Check sheet for the modelled part. Datum: model origin and axes. Units: mm. Face numbers are marked on the shaded views. A direction names the side the tool comes from. Coordinates: 2 decimals unless noted, no trailing zeros. Order: outer loops, then holes, each group sorted by start corner. A loop starts at its lowest first (then second) coordinate and runs counter-clockwise, first axis right, second up.
1. Cross-section at B-B (z = 8.5). Enter the section's corners in (x, y).
2. Cross-section at A-A (z = 43.5). Enter the section's corners in (x, y), then the cut area to 3 significant figures.
3. Thickness scan on line 1 (X direction, y = 0, z = 46.75); line 2 (Y direction, x = 0, z = 48.5); line 3 (Z direction, x = 1.2, y = 2.25). Record the ranges inside material, lowest first.
4. Set-up check for the marked faces 1 and 2: record each of +Z, -Z, +X, -X, +Y, -Y from which the full face is reachable in a straight line by a thin tool's end or side.
5. Gauge pin test, flat ends, axial feed: pin 1 Ø1.5 at (x, y) = (0, 0) entering from +Z; pin 2 Ø1 at (y, z) = (1.5, 9) entering from +X. Record the tip position at first contact, or that the pin passes through.
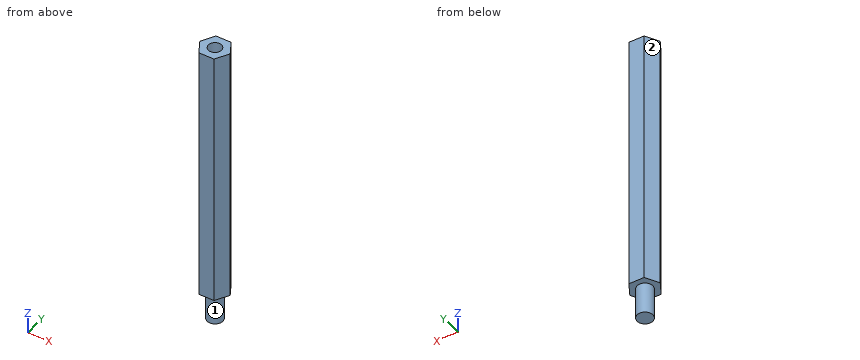
```python
from build123d import *

# Parameters (mm, degrees)
EXTRUDE_1_DEPTH = 50
SKETCH_4_R      = 1.5
EXTRUDE_2_DEPTH = 6
M3X0_5_1_D      = 2.5
M3X0_5_1_DEPTH  = 7.5
M3X0_5_1_TIP    = 0.751075774


with BuildPart() as part:
    # 草圖1 → 填料-伸長1 (new body)
    with BuildSketch(Plane.XY):
        Polygon((-1.443375673, 2.5), (-2.886751346, 0), (-1.443375673, -2.5), (1.443375673, -2.5), (2.886751346, 0), (1.443375673, 2.5), align=None)
    extrude(amount=EXTRUDE_1_DEPTH)

    # 草圖4 → 填料-伸長2 (add)
    with BuildSketch(Plane(origin=(0, 0, 0), x_dir=(-1, 0, 0), z_dir=(0, 0, -1))):
        Circle(SKETCH_4_R)
    extrude(amount=EXTRUDE_2_DEPTH)

    # M3x0.5 螺紋孔1
    with Locations(Plane.XY.offset(50)):
        with Locations((0, 0)):
            Hole(M3X0_5_1_D / 2, depth=M3X0_5_1_DEPTH)
            with Locations((0, 0, -(M3X0_5_1_DEPTH + M3X0_5_1_TIP / 2))):  # 118° drill point
                Cone(0, M3X0_5_1_D / 2, M3X0_5_1_TIP, mode=Mode.SUBTRACT)


solid = part.part
```
Data:
1. outline: (-2.89, 0) - (-1.44, -2.5) - (1.44, -2.5) - (2.89, 0) - (1.44, 2.5) - (-1.44, 2.5) - close
2. outline: (-2.89, 0) - (-1.44, -2.5) - (1.44, -2.5) - (2.89, 0) - (1.44, 2.5) - (-1.44, 2.5) - close; hole circle Ø2.5 at (0, 0)
2. area: 16.7 mm2
3. line 1: x = -2.89 to -1.25, 1.25 to 2.89
3. line 2: y = -2.5 to -1.25, 1.25 to 2.5
3. line 3: z = 0 to 50
4. face 1: -Z
4. face 2: +Z, -Z, -X, +Y
5. pin 1: stops at z = 42.2
5. pin 2: stops at x = 2.31
